Source: CAD feature listing. Evaluate the final solid. Frame: model axes, mm. A direction names the side the tool comes from. Coordinates: 2 decimals unless noted, no trailing zeros. Order: outer loops, then holes, each group sorted by start corner. A loop starts at its lowest first (then second) coordinate and runs counter-clockwise, first axis right, second up.
Autodesk Inventor part; units mm, degrees
ref_plane "YZ Plane" through (0, 0, 0) normal (1, 0, 0) x (0, 1, 0)
ref_plane "XZ Plane" through (0, 0, 0) normal (0, 1, 0) x (-1, 0, 0)
ref_plane "XY Plane" through (0, 0, 0) normal (0, 0, 1) x (1, 0, 0)
sketch "Sketch1" plane through (0, 0, 0) normal (0, 0, 1) x (1, 0, 0)
  circle A0 centre (0, 0) radius 57.5
  circle A1 centre (0, 0) radius 60.5
  line L0 (0, 0) -> (-45, -40.4382)
  line L1 (0, 0) -> (0, 20.5864)
  line L2 (0, 0) -> (45, -40.4382)
  circle A2 centre (0, 0) radius 65.5
  line L3 (-45, -40.4382) -> (-48.719, -43.7802)
  line L4 (45, -40.4382) -> (48.719, -43.7802)
  line L5 (-4.7542, 3.7944) -> (-49.0104, -35.9754)
  line L6 (-49.0104, -35.9754) -> (-65.4381, -50.7378)
  line L7 (-48.719, -43.7802) -> (-61.4277, -55.2006)
  line L8 (-65.4381, -50.7378) -> (-61.4277, -55.2006)
  arc A3 (-43.6644, -48.8229) -> (-54.3446, -48.8356) centre (-48.9974, -54.786) ccw
  line L9 (49.0104, -35.9754) -> (65.4381, -50.7378)
  line L10 (48.719, -43.7802) -> (61.4277, -55.2006)
  line L11 (65.4381, -50.7378) -> (61.4277, -55.2006)
  arc A4 (54.3446, -48.8356) -> (43.6644, -48.8229) centre (48.9974, -54.786) ccw
  line L12 (4.7542, 3.7944) -> (49.0104, -35.9754)
  point P0 (45, -40.4382)
  point P1 (42.7686, -38.433)
  point P2 (-42.7686, -38.433)
  point P3 (-46.5455, -33.7604)
  point P4 (52.5246, -39.1333)
  point P5 (43.6644, -48.8229)
  point P6 (-48.7886, -35.7761)
  point P7 (48.7886, -35.7761)
  dimension "d0" = 115
  dimension "d1" = 3
  dimension "d2" = 90
  dimension "d5" = 5
  dimension "d6" = 6
  dimension "d7" = 25.4
  dimension "d8" = 8
extrude "Extrusion1" add sketch "Sketch1" along normal mid plane 25.4 contours A1 L3 A2 L6 L5 | L12 L9 A2 L4 A1 | A1 L4 A2 L3 | L7 L8 L6 A2 | A2 A3 L7 | L10 A4 A2 | A2 L9 L11 L10
fillet "Fillet1" radius 5 4 edges at (-63.4329, -52.9692, 12.7) (-63.4329, -52.9692, -12.7) (63.4329, -52.9692, 12.7) (63.4329, -52.9692, -12.7)
sketch "Sketch2" plane through (-54.3446, -48.8356, -12.7) normal (0.6684, -0.7438, 0) x (0.7438, 0.6684, 0)
  arc A0 (-9.5228, 5) -> (-4.5228, 0) centre (-4.5228, 5) ccw
  line L0 (0, 0) -> (-4.5228, 0)
  line L1 (0, 0) -> (0, 25.4)
  line L2 (-4.5228, 25.4) -> (0, 25.4)
  arc A1 (-4.5228, 25.4) -> (-9.5228, 20.4) centre (-4.5228, 20.4) ccw
  line L3 (-9.5228, 5) -> (-9.5228, 20.4)
  line L4 (7.9525, 0) -> (7.9525, 25.4)
  line L5 (0, 25.4) -> (7.9525, 25.4)
  line L6 (0, 0) -> (0, 25.4)
  line L7 (7.9525, 0) -> (0, 0)
  circle A2 centre (0.4772, 19.4) radius 2.15
  line L8 (-9.5228, 12.7) -> (-3.8871, 12.7)
  circle A3 centre (0.4772, 6) radius 2.15
  point P0 (73.0633, 12.7)
  point P1 (0, 21.4964)
  point P2 (0, 17.3036)
  dimension "d10" = 4.3
  dimension "d11" = 10
  dimension "d17" = 6
extrude "Extrusion2" cut sketch "Sketch2" along normal through all both and the other way through all contours A3 L1 | L1 A3 | A2 L1 | L1 A2
sketch "Sketch3" plane through (-61.4277, -55.2006, -7.7) normal (0.6684, -0.7438, 0) x (0.7438, 0.6684, 0)
  arc A0 (9.5228, 16.4964) -> (9.5228, 12.3036) centre (10, 14.4) ccw
  line L0 (9.5228, 16.4964) -> (9.5228, 20.4)
  line L1 (5, 20.4) -> (9.5228, 20.4)
  arc A1 (5, 20.4) -> (0, 15.4) centre (5, 15.4) ccw
  line L2 (0, 0) -> (0, 15.4)
  arc A2 (0, 0) -> (5, -5) centre (5, 0) ccw
  line L3 (9.5228, -5) -> (5, -5)
  line L4 (9.5228, -5) -> (9.5228, -1.0964)
  circle A3 centre (10, 14.4) radius 4
  arc A4 (9.5228, 3.0964) -> (9.5228, -1.0964) centre (10, 1) ccw
  line L5 (9.5228, 3.0964) -> (9.5228, 12.3036)
  circle A5 centre (10, 1) radius 4
  point P0 (82.5861, 7.7)
  dimension "d14" = 8
extrude "Extrusion3" cut sketch "Sketch3" along normal mid plane 6 contours L0 A3 L5 A0 | A0 L5 A3 L0 | A5 L4 A4 L5 | L5 A4 L4 A5
mirror "Mirror2" about plane through (0, 0, 0) normal (1, 0, 0) of "Extrusion3", "Extrusion2"
sketch "Sketch4" plane through (0, 0, 12.7) normal (0, 0, 1) x (1, 0, 0)
  line L0 (61.7191, -47.3958) -> (57.7087, -51.8586)
  line L1 (61.7191, -47.3958) -> (48.7886, -35.7761)
  arc A0 (-48.7886, -35.7761) -> (48.7886, -35.7761) centre (0, 0) ccw
  line L2 (-48.7886, -35.7761) -> (-61.7191, -47.3958)
  line L3 (-57.7087, -51.8586) -> (-61.7191, -47.3958)
  line L4 (-57.7087, -51.8586) -> (-54.3446, -48.8356)
  arc A1 (-43.6644, -48.8229) -> (-54.3446, -48.8356) centre (-48.9974, -54.786) ccw
  arc A2 (-43.6644, -48.8229) -> (43.6644, -48.8229) centre (0, 0) ccw
  arc A3 (54.3446, -48.8356) -> (43.6644, -48.8229) centre (48.9974, -54.786) ccw
  line L5 (54.3446, -48.8356) -> (57.7087, -51.8586)
  line L6 (29.9128, -52.5878) -> (32.3849, -56.9339)
  line L7 (-61.4277, -55.2006) -> (-57.7087, -51.8586)
  line L8 (-57.7087, -51.8586) -> (-61.7191, -47.3958)
  line L9 (-61.7191, -47.3958) -> (-65.4381, -50.7378)
  line L10 (-65.4381, -50.7378) -> (-61.4277, -55.2006)
extrude "Extrusion4" cut sketch "Sketch4" against normal through all contours L6 A2 A1 L4 L3 L2 A0 | L3 L7 L10 L9
properties part number "CANALETA_MOVIL" material "Steel, Mild, Welded"
1. Access query for faces 4 (the face through (38.32, -53.12, -0.18)), 5 (the face through (57.277, -47.435, -8.422)), 6 (the face through (63.46, -52.94, -0.11)). Directions: +Z, -Z, +X, -X, +Y, -Y. A direction counts if a zero-diameter tool reaches every point of the face in a straight line with its end or side. Return the directions, or none.
Findings:
face 4: +Z, -Z, -Y
face 5: none
face 6: +Z, -Z, +X, -Y
2. Ray query, line 1 (Y direction, x = 56, z = 10); line 2 (X direction, y = -52, z = -3.75); line 3 (X direction, y = -52.75, z = 2.75). Return the intervals inside material, ascending.
Findings:
line 1: y = -50.32 to -49.66, -46.29 to -42.26
line 2: x = 30.92 to 39.83, 57.87 to 64.3
line 3: x = 30.01 to 38.83, 58.7 to 63.63
3. Draft query along X for faces 1 (the face through (62.29, -52, -11.27)), 2 (the face through (40.37, -45.06, -0.18)), 3 (the face through (52.04, -44.98, 7.9)). Return one class per face: released by +X, released by -X, zero draft, split by the parting line, or undercut.
Findings:
face 1: released by +X
face 2: released by -X
face 3: undercut
4. Section query D-D on y = -46. Count the separate pieces of the cut face and the enclosed holes in it, plus the area to 3 significant figures.
Findings:
separate pieces: 1
enclosed holes: 2
area: 447 mm2
5. Section query C-C on y = -39.5. Return loops of the section in (x, z).
Findings:
outline: (45.83, -12.7) - (52.93, -12.7) - (52.93, 12.7) - (45.83, 12.7) - close
6. Pin query (flat end, axial travel): P1, Ø3, axis at y = -38, z = -1, coming from the -X side; P2, Ø2, axis at x = 55, z = 3.5, coming from the -Y side; P3, Ø12, axis at x = 46, z = 5, coming from the -Y side. Return the tip coordinate at first contact, or that it passes through.
Findings:
P1: stops at x = 45.83
P2: stops at y = -50.32
P3: stops at y = -51.87
7. Section query B-B on x = 47. Return loops of the section in (y, z).
Findings:
outline: (-47.04, -12.7) - (-38.1, -12.7) - (-38.1, 12.7) - (-47.04, 12.7) - close
8. Section query A-A on z = 5. Return loops of the section in (x, y), plus the area to 3 significant figures.
Findings:
outline: (29.91, -52.59) - (32.38, -56.93) arc R65.5 ccw to (43.66, -48.82) arc R8 cw to (50.54, -46.94) - (53.3, -43.86) - (55.02, -45.4) - (57.02, -43.17) - (49.01, -35.98) - (48.79, -35.78) arc R60.5 cw to start; (56.68, -50.94) - (61.43, -55.2) - (65.44, -50.74) - (58.98, -44.93) - (56.98, -47.16) - (58.69, -48.7) - close
area: 215 mm2
